```python
from build123d import *

# Parameters (mm, degrees)
SKETCH1_W                = 159.078855478
SKETCH1_H                = 159.078855478
BOSS_EXTRUDE1_DEPTH      = 101.6
BOSS_EXTRUDE1_DEPTH_BACK = 50.8
BOSS_EXTRUDE3_START      = 101.6
SKETCH1_5_R              = 11.43
BOSS_EXTRUDE3_DEPTH      = 5.08
SKETCH3_R                = 1.6
CUT_EXTRUDE1_DEPTH       = 202.510224058
FILLET4_R                = 5.08
SKETCH4_R                = 2.1
CUT_EXTRUDE2_DEPTH       = 5.08
SKETCH5_R                = 3.5
SKETCH5_R_2              = 5.207
SKETCH5_R_3              = 1.65
SKETCH5_W                = 19
SKETCH5_H                = 12.5
SKETCH5_W_2              = 18.7
SKETCH5_H_2              = 23.3
CUT_EXTRUDE3_DEPTH       = 9.360572261
SKETCH7_W                = 25.4
SKETCH7_H                = 5.08
CUT_EXTRUDE4_DEPTH       = 5.588
BOSS_EXTRUDE4_DEPTH      = 25.4
CUT_EXTRUDE5_DEPTH       = 25.4
SKETCH11_W               = 12.7
SKETCH11_H               = 4.572
CUT_EXTRUDE6_DEPTH       = 5.334
CUT_EXTRUDE7_DEPTH       = 2.54
CUT_EXTRUDE8_DEPTH       = 16.764
SKETCH13_R               = 6.5
CUT_EXTRUDE9_DEPTH       = 5.08


with BuildPart() as part:
    # Sketch1 → Boss-Extrude1 (new, two sides)
    with BuildSketch(Plane(origin=(0, 0, 0), x_dir=(1, 0, 0), z_dir=(0, 1, 0))) as boss_extrude1_sk:
        with BuildLine():
            Line((-83.82, -88.9), (83.82, -88.9))
            ThreePointArc((83.82, -88.9), (87.412102448, -87.412102448), (88.9, -83.82))
            Line((88.9, -83.82), (88.9, 83.82))
            ThreePointArc((88.9, 83.82), (87.412102448, 87.412102448), (83.82, 88.9))
            Line((83.82, 88.9), (-83.82, 88.9))
            ThreePointArc((-83.82, 88.9), (-87.412102448, 87.412102448), (-88.9, 83.82))
            Line((-88.9, 83.82), (-88.9, -83.82))
            ThreePointArc((-88.9, -83.82), (-87.412102448, -87.412102448), (-83.82, -88.9))
        make_face()
        Rectangle(SKETCH1_W, SKETCH1_H, mode=Mode.SUBTRACT)
    extrude(amount=BOSS_EXTRUDE1_DEPTH)
    extrude(boss_extrude1_sk.sketch, amount=-BOSS_EXTRUDE1_DEPTH_BACK)

    # Sketch1<5> → Boss-Extrude3 (add)
    with BuildSketch(Plane(origin=(0, 0, 0), x_dir=(1, 0, 0), z_dir=(0, 1, 0)).offset(BOSS_EXTRUDE3_START)):
        with BuildLine():
            ThreePointArc((-88.9, -83.82), (-87.412102448, -87.412102448), (-83.82, -88.9))
            Line((-83.82, -88.9), (83.82, -88.9))
            ThreePointArc((83.82, -88.9), (87.412102448, -87.412102448), (88.9, -83.82))
            Line((88.9, -83.82), (88.9, 83.82))
            ThreePointArc((88.9, 83.82), (87.412102448, 87.412102448), (83.82, 88.9))
            Line((83.82, 88.9), (-83.82, 88.9))
            ThreePointArc((-83.82, 88.9), (-87.412102448, 87.412102448), (-88.9, 83.82))
            Line((-88.9, 83.82), (-88.9, -83.82))
        make_face()
        with Locations(Location((0, 0, 0), (0, 0, 270))):
            Circle(SKETCH1_5_R, mode=Mode.SUBTRACT)
    extrude(amount=BOSS_EXTRUDE3_DEPTH)

    # Sketch3 → Cut-Extrude1 (cut, through all)
    with BuildSketch(Plane(origin=(0, 106.68, 0), x_dir=(1, 0, 0), z_dir=(0, 1, 0))):
        with Locations(Location((-15.5, 15.5, 0), (0, 0, 270))):
            Circle(SKETCH3_R)
        with Locations(Location((-15.5, -15.5, 0), (0, 0, 270))):
            Circle(SKETCH3_R)
        with Locations(Location((15.5, 15.5, 0), (0, 0, 270))):
            Circle(SKETCH3_R)
        with Locations(Location((15.5, -15.5, 0), (0, 0, 270))):
            Circle(SKETCH3_R)
    extrude(amount=-CUT_EXTRUDE1_DEPTH, mode=Mode.SUBTRACT)

    # Fillet4
    fillet4_edges = [part.edges().sort_by_distance(p)[0] for p in [
        (79.539427739, 25.4, -79.539427739),
        (-79.539427739, 25.4, -79.539427739),
        (-79.539427739, 25.4, 79.539427739),
        (79.539427739, 25.4, 79.539427739),
    ]]
    fillet(fillet4_edges, radius=FILLET4_R)

    # Sketch4 → Cut-Extrude2 (cut)
    with BuildSketch(Plane(origin=(0, 106.68, 0), x_dir=(1, 0, 0), z_dir=(0, 1, 0))):
        with Locations(Location((-40.66, 40.66, 0), (0, 0, 270))):
            Circle(SKETCH4_R)
        with Locations(Location((40.66, 40.66, 0), (0, 0, 270))):
            Circle(SKETCH4_R)
        with Locations(Location((-40.66, -40.66, 0), (0, 0, 270))):
            Circle(SKETCH4_R)
        with Locations(Location((40.66, -40.66, 0), (0, 0, 270))):
            Circle(SKETCH4_R)
    extrude(amount=-CUT_EXTRUDE2_DEPTH, mode=Mode.SUBTRACT)

    # Sketch5 → Cut-Extrude3 (cut)
    with BuildSketch(Plane.XY.offset(88.9)):
        with Locations((-34.158642562, -11.51833892)):
            Circle(SKETCH5_R)
        with Locations((-55.102312512, -31.62532479)):
            Circle(SKETCH5_R_2)
        with Locations((-13.97, 15.0114)):
            Circle(SKETCH5_R_3)
        with Locations((-13.97, -15.0114)):
            Circle(SKETCH5_R_3)
        with Locations((-55.584910431, -11.51833892)):
            Rectangle(SKETCH5_W, SKETCH5_H)
        with Locations((-13.97, 0)):
            Rectangle(SKETCH5_W_2, SKETCH5_H_2)
    extrude(amount=-CUT_EXTRUDE3_DEPTH, mode=Mode.SUBTRACT)

    # Sketch7 → Cut-Extrude4 (cut)
    with BuildSketch(Plane.XZ.offset(50.8)):
        with Locations((0, -82.079427739)):
            Rectangle(SKETCH7_W, SKETCH7_H)
    extrude(amount=-CUT_EXTRUDE4_DEPTH, mode=Mode.SUBTRACT)

    # Sketch10 → Boss-Extrude4 (add)
    with BuildSketch(Plane.ZY.offset(-12.7)):
        Polygon((-79.539427739, -38.354), (-79.539427739, -41.148), (-81.063427739, -41.148), align=None)
    extrude(amount=BOSS_EXTRUDE4_DEPTH)

    # Sketch10<2> → Cut-Extrude5 (cut)
    with BuildSketch(Plane.ZY.offset(-12.7)):
        Polygon((-79.539427739, -38.354), (-79.539427739, -41.148), (-81.063427739, -41.148), align=None)
    extrude(amount=CUT_EXTRUDE5_DEPTH, mode=Mode.SUBTRACT)

    # Sketch11 → Cut-Extrude6 (cut)
    with BuildSketch(Plane(origin=(0, 0, 79.539427739), x_dir=(-1, 0, 0), z_dir=(0, 0, -1))):
        with Locations((-44.45, -43.434)):
            Rectangle(SKETCH11_W, SKETCH11_H)
        with Locations((44.45, -43.434)):
            Rectangle(SKETCH11_W, SKETCH11_H)
    extrude(amount=-CUT_EXTRUDE6_DEPTH, mode=Mode.SUBTRACT)

    # Sketch12 → Cut-Extrude7 (cut)
    with BuildSketch(Plane(origin=(0, 106.68, 0), x_dir=(1, 0, 0), z_dir=(0, 1, 0))):
        with BuildLine():
            Line((38.210330331, 70.326189438), (66.435994121, 70.326189438))
            ThreePointArc((66.435994121, 70.326189438), (71.515994121, 65.246189438), (66.435994121, 60.166189438))
            Line((66.435994121, 60.166189438), (38.210330331, 60.166189438))
            ThreePointArc((38.210330331, 60.166189438), (33.130330331, 65.246189438), (38.210330331, 70.326189438))
        make_face()
    extrude(amount=-CUT_EXTRUDE7_DEPTH, mode=Mode.SUBTRACT)

    # Sketch12<2> → Cut-Extrude8 (cut)
    with BuildSketch(Plane(origin=(0, 106.68, 0), x_dir=(1, 0, 0), z_dir=(0, 1, 0))):
        with BuildLine():
            Line((38.210330331, 70.326189438), (66.435994121, 70.326189438))
            ThreePointArc((66.435994121, 70.326189438), (71.515994121, 65.246189438), (66.435994121, 60.166189438))
            Line((66.435994121, 60.166189438), (38.210330331, 60.166189438))
            ThreePointArc((38.210330331, 60.166189438), (33.130330331, 65.246189438), (38.210330331, 70.326189438))
        make_face()
    extrude(amount=-CUT_EXTRUDE8_DEPTH, mode=Mode.SUBTRACT)

    # Sketch13 → Cut-Extrude9 (cut)
    with BuildSketch(Plane(origin=(0, 0, 79.539427739), x_dir=(-1, 0, 0), z_dir=(0, 0, -1))):
        with Locations((34.158642562, -11.51833892)):
            Circle(SKETCH13_R)
    extrude(amount=-CUT_EXTRUDE9_DEPTH, mode=Mode.SUBTRACT)


solid = part.part
```
The model under review builds one solid part; all positions refer to its coordinate system, in mm. A direction names the side the tool comes from. Round coordinates to 2 decimals unless told otherwise and drop trailing zeros. Order: outer loops, then holes, each group sorted by start corner. A loop starts at its lowest first (then second) coordinate and runs counter-clockwise, first axis right, second up. Notation, with made-up numbers: (37.5, -34) - (45.5, -34) arc R18 ccw to (45.5, -30) - close; hole circle Ø3 at (-20.5, 61.25). An arc over 180 degrees is marked (long way). Answer in a Markdown table with one row per item.
(1) For line 1 (X direction, y = 103.05, z = -15.5); line 2 (Y direction, x = -13.97, z = 85.5); line 3 (X direction, y = 64.5, z = 22), list the stretches that pass through material, from the lowest coordinate up. Write a range as from..to.
Result set:
| item | result |
|---|---|
| line 1 | x = -88.9..-17.1, -13.9..13.9, 17.1..88.9 |
| line 2 | y = -50.8..-16.66, -13.36..-11.65, 11.65..13.36, 16.66..106.68 |
| line 3 | x = -88.9..-79.54, 79.54..88.9 |
(2) Machinability: for faces 1 (the face through (-56, -17.768, 84)), 2 (the face through (52, 104, -70.326)), 3 (the face through (-50.8, -43, 82)), 4 (the face through (78, 24.3, 78.1)), which of the approach directions +Z, -Z, +X, -X, +Y, -Y give a long, thin tool a straight path to every point of the face, cutting with its end or side? Answer none if there is none.
Result set:
| item | result |
|---|---|
| face 1 | +Z |
| face 2 | +Y, -Y |
| face 3 | none |
| face 4 | -Y |
(3) Take a section at C-C on z = 4. Write out the cut boundary in (x, y), plus the area to 3 significant figures.
Result set:
| item | result |
|---|---|
| outline | (-88.9, -50.8) - (-79.54, -50.8) - (-79.54, 101.6) - (-10.71, 101.6) - (-10.71, 106.68) - (-88.9, 106.68) - close; (10.71, 101.6) - (79.54, 101.6) - (79.54, -50.8) - (88.9, -50.8) - (88.9, 106.68) - (10.71, 106.68) - close |
| area | 3,650 mm2 |
(4) Take a section at D-D on z = 51.5. Write out the cut boundary in (x, y).
Result set:
| item | result |
|---|---|
| outline | (-88.9, -50.8) - (-79.54, -50.8) - (-79.54, 101.6) - (79.54, 101.6) - (79.54, -50.8) - (88.9, -50.8) - (88.9, 106.68) - (-88.9, 106.68) - close |
(5) Take a section at B-B on x = 62. Write out the cut boundary in (y, z).
Result set:
| item | result |
|---|---|
| outline | (-50.8, -88.9) - (106.68, -88.9) - (106.68, -70.33) - (101.6, -70.33) - (101.6, -79.54) - (-50.8, -79.54) - close; (-50.8, 79.54) - (101.6, 79.54) - (101.6, -60.17) - (106.68, -60.17) - (106.68, 88.9) - (-50.8, 88.9) - close |
(6) Take a section at A-A on y = 25.5. Write out the cut boundary in (x, z).
Result set:
| item | result |
|---|---|
| outline | (-88.9, -83.82) arc R5.08 ccw to (-83.82, -88.9) - (83.82, -88.9) arc R5.08 ccw to (88.9, -83.82) - (88.9, 83.82) arc R5.08 ccw to (83.82, 88.9) - (-83.82, 88.9) arc R5.08 ccw to (-88.9, 83.82) - close; hole (-79.54, -74.46) arc R5.08 ccw to (-74.46, -79.54) - (74.46, -79.54) arc R5.08 ccw to (79.54, -74.46) - (79.54, 74.46) arc R5.08 ccw to (74.46, 79.54) - (-74.46, 79.54) arc R5.08 ccw to (-79.54, 74.46) - close |
(7) Mouldability with a two-part tool opening along Y and no side actions: class faces 5 (the face through (53, 104, -60.166)), 6 (the face through (-65.085, -12, 84)), 7 (the face through (-1, 101.6, -19)) as released by +Y, released by -Y, zero draft, split by the parting line, or undercut.
Result set:
| item | result |
|---|---|
| face 5 | zero draft |
| face 6 | undercut |
| face 7 | released by -Y |
(8) Clearance check with flat-ended pins moving along their axes: P1, Ø1.5, axis at x = 57.5, z = 25.5, coming from the -Y side; P2, Ø4.5, axis at y = -2, z = 84, coming from the -X side. State where each tip first meets the part, or that it passes through.
Result set:
| item | result |
|---|---|
| P1 | stops at y = 101.6 |
| P2 | stops at x = -88.9 |
